Input: part model. Units: mm. Frame: model coordinates. A direction names the side the tool comes from. Round coordinates to 2 decimals unless told otherwise and drop trailing zeros. Loops run counter-clockwise (first coordinate to the right, second up) from the corner with the lowest first, then second, coordinate; pieces in that order, holes last. Notation, with made-up numbers: (-35, -32.75) - (3, -32.75) arc R22 cw to (3, 5.25) - close; hole circle Ø3 at (-32.5, -20.75). An arc over 180 degrees is marked (long way). One line per question, with ' | ' between items. Start each with the question number.
Item 1: First-contact query: pin 1 (12 mm diameter, centred on x = -33, y = 61.5, fed in from +Z); pin 2 (10 mm diameter, centred on x = -46, z = 52.5, fed in from -Y); pin 3 (1 mm diameter, centred on x = -18, y = 97.5, fed in from -Z); pin 4 (1.5 mm diameter, centred on x = 3.5, z = -59.5, fed in from +Y). Flat tips, straight axial feed; report the tip coordinate or a pass-through.
Item 2: Set-up query: faces 1 (the face through (-6.881, 103.936, 6.232)), 2 (the face through (-7, 60, -5)), 3 (the face through (-1.38, 90.88, -0.07)), 4 (the face through (-2, 95, 10)), 5 (the face through (-45.636, 7.395, -59.517)). Return all of +Z, -Z, +X, -X, +Y, -Y with unobstructed straight access to the full face (end or side cutting, diameter ignored); none if empty.
Item 3: Section A-A, the plane z = 0. Return loops of the section in (x, y), plus the area to 3 significant figures.
Item 4: Draft query along X for faces 6 (the face through (-2, 96, 5)), 7 (the face through (6.33, 113.6, 0.04)), 8 (the face through (-6, 21, 7)). Return one class per face: pulls with the +X half, pulls with the -X half, needs draft (parallel to the pull), parting line crosses it, or undercut.
Item 5: Material intervals for line 1 along Z through (x, y) = (-2.5, 83); line 2 along Y through (x, z) = (6, -39); line 3 along Z through (x, y) = (-44, 12), sorted ascending.
```python
from build123d import *

# Parameters (mm, degrees)
SKETCH1_R           = 75
BOSS_EXTRUDE1_DEPTH = 20
FILLET1_R           = 5
BOSS_EXTRUDE2_DEPTH = 5
CHAMFER2_SIZE       = 2.5
CHAMFER3_SIZE       = 2.5
FILLET2_R           = 5
SKETCH3_R           = 10
BOSS_EXTRUDE4_DEPTH = 5
FILLET5_R           = 2.5
SKETCH5_R           = 5
CUT_EXTRUDE4_DEPTH  = 10


with BuildPart() as part:
    # Sketch1 → Boss-Extrude1 (new body)
    with BuildSketch(Plane(origin=(0, 0, 0), x_dir=(1, 0, 0), z_dir=(0, 1, 0))):
        with Locations(Location((0, 0, 0), (0, 0, 270))):
            Circle(SKETCH1_R)
    extrude(amount=BOSS_EXTRUDE1_DEPTH)

    # Fillet1
    fillet1_edges = [part.edges().sort_by_distance(p)[0] for p in [
        (0, 20, -75),
    ]]
    fillet(fillet1_edges, radius=FILLET1_R)

    # Sketch2 → Boss-Extrude2 (add, symmetric)
    with BuildSketch(Plane.XY):
        with BuildLine():
            Line((-35, 12.444541462), (30, 12.444541462))
            Line((30, 12.444541462), (30, 14.22534194))
            ThreePointArc((30, 14.22534194), (17.339153051, 55.705537473), (14.967295478, 99.010017132))
            ThreePointArc((14.967295478, 99.010017132), (6.101321608, 113.703060776), (-10.750360925, 110.460867076))
            ThreePointArc((-10.750360925, 110.460867076), (-36.154540949, 64.738072262), (-35, 12.444541462))
        make_face()
    extrude(amount=BOSS_EXTRUDE2_DEPTH, both=True)

    # Chamfer2
    chamfer2_edges = [part.edges().sort_by_distance(p)[0] for p in [
        (16.818841315, 58.796417799, 5),
        (6.101321608, 113.703060776, 5),
        (-35.144979175, 68.502452567, 5),
    ]]
    chamfer(chamfer2_edges, length=CHAMFER2_SIZE)

    # Chamfer3
    chamfer3_edges = [part.edges().sort_by_distance(p)[0] for p in [
        (-35.144979175, 68.502452567, -5),
        (16.818841315, 58.796417799, -5),
        (6.101321608, 113.703060776, -5),
    ]]
    chamfer(chamfer3_edges, length=CHAMFER3_SIZE)

    # Fillet2
    fillet2_edges = [part.edges().sort_by_distance(p)[0] for p in [
        (-4.741993221, 20, 5),
        (-4.741993221, 20, -5),
    ]]
    fillet(fillet2_edges, radius=FILLET2_R)

    # Sketch3 → Boss-Extrude4 (add)
    with BuildSketch(Plane.XY.offset(5)):
        with Locations(Location((-2.266839378, 95.064766839, 0), (0, 0, 180))):
            Circle(SKETCH3_R)
    extrude(amount=BOSS_EXTRUDE4_DEPTH)

    # Fillet5
    fillet5_edges = [part.edges().sort_by_distance(p)[0] for p in [
        (7.733160622, 95.064766839, 10),
    ]]
    fillet(fillet5_edges, radius=FILLET5_R)

    # Sketch5 → Cut-Extrude4 (cut)
    with BuildSketch(Plane(origin=(0, 0, -5), x_dir=(-1, 0, 0), z_dir=(0, 0, -1))):
        with Locations((2.460107282, 95.761056281)):
            Circle(SKETCH5_R)
    extrude(amount=-CUT_EXTRUDE4_DEPTH, mode=Mode.SUBTRACT)


solid = part.part
```
Return value:
1) pin 1: z = 5 | pin 2: y = 0 | pin 3: z = -5 | pin 4: y = 20
2) face 1: +Z | face 2: -Z, +X, -X, +Y | face 3: -Z | face 4: +Z, +X, -X, +Y | face 5: +Y, -Y
3) outline: (-75, 0) - (75, 0) - (75, 15) arc R5 ccw to (70, 20) - (27.56, 20) arc R180 cw to (14.97, 99.01) arc R15 ccw to (-10.75, 110.46) arc R100 ccw to (-36.91, 20) - (-70, 20) arc R5 ccw to (-75, 15) - close; hole circle Ø10 at (-2.46, 95.76) | area: 7,480 mm2
4) face 6: undercut | face 7: parting line crosses it | face 8: needs draft
5) line 1: -5 to 5 | line 2: 0 to 20 | line 3: -60.74 to 60.74
